from build123d import *

# Parameters (mm, degrees)
ESQUISSE2_W             = 65
ESQUISSE2_H             = 14
BOSS_EXTRU_1_DEPTH      = 4
ESQUISSE3_R             = 5.5
ESQUISSE3_R_2           = 1.5
ENL_V_MAT_EXTRU_1_DEPTH = 4
BOSS_EXTRU_3_DEPTH      = 14
ESQUISSE7_R             = 12.5
ENL_V_MAT_EXTRU_4_DEPTH = 39.788005272
CHANFREIN1_SIZE         = 4
CHANFREIN2_SIZE         = 1


with BuildPart() as part:
    # Esquisse2 → Boss.-Extru.1 (new body)
    with BuildSketch(Plane(origin=(0, 0, 0), x_dir=(1, 0, 0), z_dir=(0, 1, 0))):
        with Locations((-3.326098768, -2.352831094)):
            Rectangle(ESQUISSE2_W, ESQUISSE2_H)
    extrude(amount=-BOSS_EXTRU_1_DEPTH)

    # Esquisse3 → Enlèv. mat.-Extru.1 (cut)
    with BuildSketch(Plane.XZ.offset(4)):
        with Locations(Location((-28.826098768, 2.352831094, 0), (0, 0, 270))):
            Circle(ESQUISSE3_R)
        with Locations(Location((22.173901232, 2.352831094, 0), (0, 0, 270))):
            Circle(ESQUISSE3_R)
        with Locations(Location((-20.326098768, 2.352831094, 0), (0, 0, 270))):
            Circle(ESQUISSE3_R_2)
        with Locations(Location((13.673901232, 2.352831094, 0), (0, 0, 270))):
            Circle(ESQUISSE3_R_2)
    extrude(amount=-ENL_V_MAT_EXTRU_1_DEPTH, mode=Mode.SUBTRACT)

    # Esquisse5 → Boss.-Extru.3 (add)
    with BuildSketch(Plane(origin=(0, 0, -4.647168906), x_dir=(-1, 0, 0), z_dir=(0, 0, -1))):
        with BuildLine():
            Line((-10.421628317, -4), (17.073825853, -4))
            ThreePointArc((17.073825853, -4), (3.326098768, 5), (-10.421628317, -4))
        make_face()
    extrude(amount=-BOSS_EXTRU_3_DEPTH)

    # Esquisse7 → Enlèv. mat.-Extru.4 (cut, through all)
    with BuildSketch(Plane(origin=(0, 0, -4.647168906), x_dir=(-1, 0, 0), z_dir=(0, 0, -1))):
        with Locations((3.326098768, -10)):
            Circle(ESQUISSE7_R)
    extrude(amount=-ENL_V_MAT_EXTRU_4_DEPTH, mode=Mode.SUBTRACT)

    # Chanfrein1
    chanfrein1_edges = [part.edges().sort_by_distance(p)[0] for p in [
        (-35.826098768, -2, -4.647168906),
        (29.173901232, -2, -4.647168906),
        (29.173901232, -2, 9.352831094),
        (-35.826098768, -2, 9.352831094),
    ]]
    chamfer(chanfrein1_edges, length=CHANFREIN1_SIZE)

    # Chanfrein2
    chanfrein2_edges = [part.edges().sort_by_distance(p)[0] for p in [
        (-3.326098768, 5, 9.352831094),
        (-3.326098768, 5, -4.647168906),
    ]]
    chamfer(chanfrein2_edges, length=CHANFREIN2_SIZE)


solid = part.part
CAD build for the part. Positions are in the model's coordinates, mm. Round coordinates to 2 decimals unless told otherwise and drop trailing zeros. Loops run counter-clockwise (first coordinate to the right, second up) from the corner with the lowest first, then second, coordinate; pieces in that order, holes last. Notation, with made-up numbers: (47, 0.5) - (52, 0.5) arc R28 cw to (52, 31.5) - close; hole circle Ø3 at (18.5, 30.5). An arc over 180 degrees is marked (long way). Put each result on its own line as item: value.
1. Wall check: line 1 (X direction, y = -2, z = 0.25); line 2 (X direction, y = -1.25, z = 6.5); line 3 (Z direction, x = 22, y = -1.25). Give the ranges that are in metal, low to high.
Geometry check:
line 1: -35.83 to -33.91, -23.74 to -12.93, 6.28 to 17.09, 27.26 to 29.17
line 2: -34.68 to -32.44, -25.21 to -12.25, 5.6 to 18.56, 25.79 to 28.03
line 3: -4.65 to -3.14, 7.85 to 9.35
2. Slice it at C-C on x = 20. List the corners of the cut face in (y, z), and give its area (3 significant figures).
Geometry check:
outline: (-4, -4.65) - (0, -4.65) - (0, -2.7) - (-4, -2.7) - close; (-4, 7.4) - (0, 7.4) - (0, 9.35) - (-4, 9.35) - close
area: 15.6 mm²
3. Slice it at D-D on z = -1.5. List the corners of the cut face in (x, y), and give its area (3 significant figures).
Geometry check:
outline: (-34.97, -4) - (-32.75, -4) - (-32.75, 0) - (-34.97, 0) - close; (-24.9, -4) - (-14.29, -4) arc R12.5 cw to (7.64, -4) - (18.25, -4) - (18.25, 0) - (7.85, 0) arc R15 ccw to (-14.51, 0) - (-24.9, 0) - close; (26.1, -4) - (28.32, -4) - (28.32, 0) - (26.1, 0) - close
area: 166 mm²
4. Two-plate mould, pull along X, no slides. Class faces 1 (the flat face through (16, -4, 2)), 2 (the cylindrical face through (-33.7, -2, -0.2)), 3 (the flat face through (-33.854, -1.972, 7.325)): released by +X, released by -X, zero draft, split by the parting line, or undercut.
Geometry check:
face 1: zero draft
face 2: undercut
face 3: released by -X
5. Slice it at A-A on y = -3.25. List the corners of the cut face in (x, z), and give its area (3 significant figures).
Geometry check:
outline: (-35.83, -0.65) - (-31.83, -4.65) - (-13.85, -4.65) - (-13.85, 9.35) - (-31.83, 9.35) - (-35.83, 5.35) - close; (7.19, -4.65) - (25.17, -4.65) - (29.17, -0.65) - (29.17, 5.35) - (25.17, 9.35) - (7.19, 9.35) - close; hole circle Ø11 at (-28.83, 2.35); hole circle Ø3 at (-20.33, 2.35); hole circle Ø3 at (13.67, 2.35); hole circle Ø11 at (22.17, 2.35)
area: 379 mm²
6. Slice it at B-B on z = 3. List the corners of the cut face in (x, y), and give its area (3 significant figures).
Geometry check:
outline: (-35.83, -4) - (-34.29, -4) - (-34.29, 0) - (-35.83, 0) - close; (-23.36, -4) - (-21.68, -4) - (-21.68, 0) - (-23.36, 0) - close; (-18.97, -4) - (-14.29, -4) arc R12.5 cw to (7.64, -4) - (12.32, -4) - (12.32, 0) - (7.85, 0) arc R15 ccw to (-14.51, 0) - (-18.97, 0) - close; (15.03, -4) - (16.71, -4) - (16.71, 0) - (15.03, 0) - close; (27.64, -4) - (29.17, -4) - (29.17, 0) - (27.64, 0) - close
area: 127 mm²
7. Pin check, flat tips, straight feed: P1, Ø4, axis at y = 3, z = 3, coming from the -X side; P2, Ø2, axis at x = -7.5, y = 0, coming from the +Z side; P3, Ø4, axis at x = 8, y = 2.5, coming from the +Z side. Stop position of each tip, or through.
Geometry check:
P1: x = -13.52
P2: through
P3: z = 8.48
